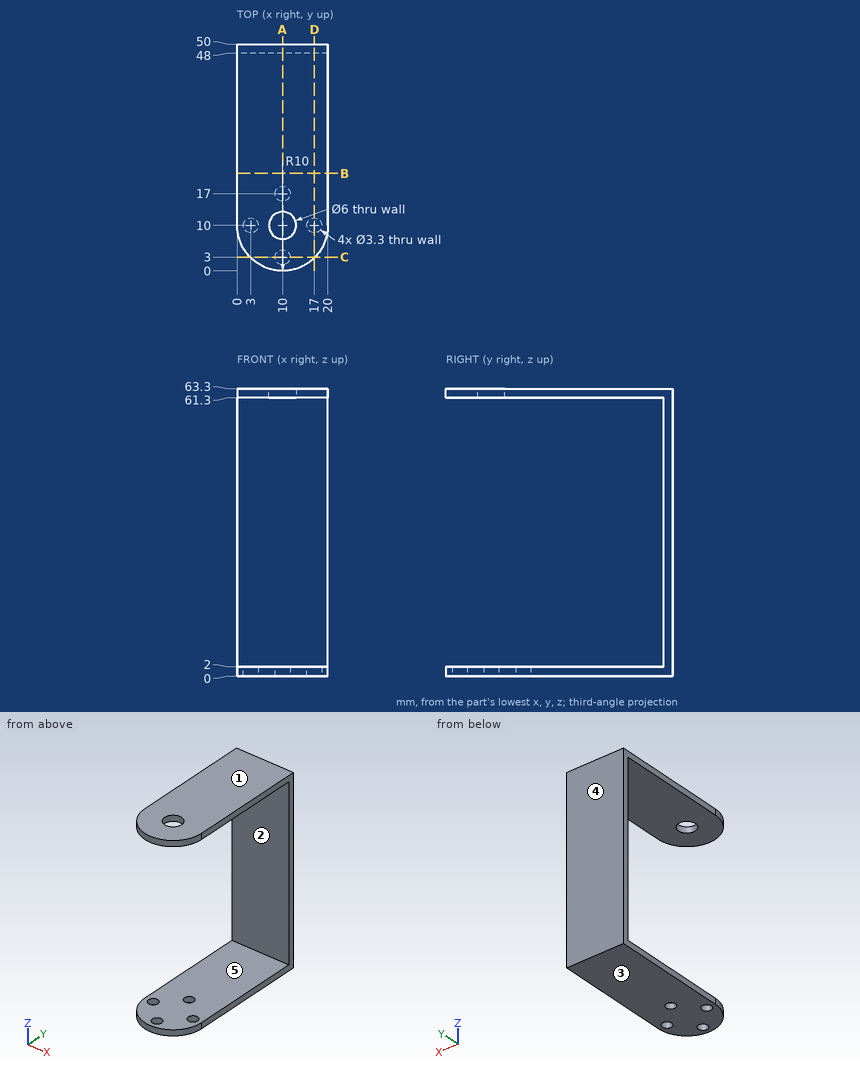
Geometry: see drawing. Coordinates: mm, zero at the bounding-box minimum. A direction names the side the tool comes from. Coordinates: 2 decimals unless noted, no trailing zeros. Order: outer loops, then holes, each group sorted by start corner. A loop starts at its lowest first (then second) coordinate and runs counter-clockwise, first axis right, second up. Notation, with made-up numbers: (75, 81) - (114, 81) arc R25 ccw to (114, 97) - close; hole circle Ø3 at (-31, -38.5). An arc over 180 degrees is marked (long way). Return JSON: item names as keys, results as strings.
Q1. Access query for the marked faces 1 and 2. Directions: +Z, -Z, +X, -X, +Y, -Y. A direction counts if a zero-diameter tool reaches every point of the face in a straight line with its end or side. Return the directions, or none.
The answers:
{"face 1": "+Z, +X, -X, +Y, -Y", "face 2": "+X, -X, -Y"}
Q2. Ray query, probe 1 along Z at (x, y) = (13.25, 13.5); probe 2 along Y at (x, z) = (7.5, 36.5); probe 3 along Z at (x, y) = (7.5, 10.5). Return the intervals inside material, ascending.
The answers:
{"probe 1": "z = 0 to 2, 61.3 to 63.3", "probe 2": "y = 48 to 50", "probe 3": "z = 0 to 2"}
Q3. Cut plane D-D (x = 17). Return loops of the section in (y, z), then the cut area to 3 significant figures.
The answers:
{"outline": "(2.86, 0) - (8.35, 0) - (8.35, 2) - (2.86, 2) - close; (2.86, 61.3) - (48, 61.3) - (48, 2) - (11.65, 2) - (11.65, 0) - (50, 0) - (50, 63.3) - (2.86, 63.3) - close", "area": "301 mm2"}
Q4. Cut plane A-A (x = 10). Return loops of the section in (y, z), then the cut area to 3 significant figures.
The answers:
{"outline": "(0, 0) - (1.35, 0) - (1.35, 2) - (0, 2) - close; (0, 61.3) - (7, 61.3) - (7, 63.3) - (0, 63.3) - close; (4.65, 0) - (15.35, 0) - (15.35, 2) - (4.65, 2) - close; (13, 61.3) - (48, 61.3) - (48, 2) - (18.65, 2) - (18.65, 0) - (50, 0) - (50, 63.3) - (13, 63.3) - close", "area": "293 mm2"}
Q5. Draft query along Z for the marked faces 3, 4 and 5. Return one class per face: +Z half, -Z half, draft (parallel to the pull), parting line (faces both ways), or undercut.
The answers:
{"face 3": "-Z half", "face 4": "draft", "face 5": "undercut"}
Q6. Cut plane C-C (y = 3). Return loops of the section in (x, z), then the cut area to 3 significant figures.
The answers:
{"outline": "(2.86, 0) - (8.35, 0) - (8.35, 2) - (2.86, 2) - close; (2.86, 61.3) - (17.14, 61.3) - (17.14, 63.3) - (2.86, 63.3) - close; (11.65, 0) - (17.14, 0) - (17.14, 2) - (11.65, 2) - close", "area": "50.5 mm2"}
Q7. Cut plane B-B (y = 21.5). Return loops of the section in (x, z).
The answers:
{"outline": "(0, 0) - (20, 0) - (20, 2) - (0, 2) - close; (0, 61.3) - (20, 61.3) - (20, 63.3) - (0, 63.3) - close"}
Q8. First-contact query: pin 1 (3 mm diameter, centred on x = 17, y = 10, fed in from -Z); pin 2 (8 mm diameter, centred on x = 15.5, z = 24.5, fed in from -Y); pin 3 (9.5 mm diameter, centred on x = 10, y = 10, fed in from -Z). Flat tips, straight axial feed; report the tip coordinate or a pass-through.
The answers:
{"pin 1": "stops at z = 61.3", "pin 2": "stops at y = 48", "pin 3": "stops at z = 0"}
